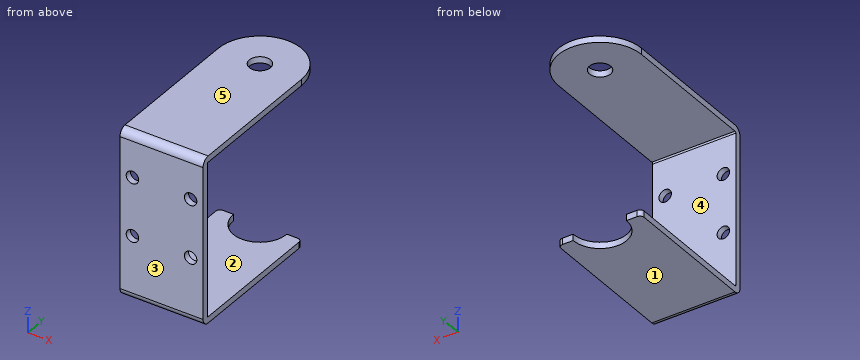
Autodesk Inventor part; units mm, degrees
ref_plane "YZ Plane" through (0, 0, 0) normal (1, 0, 0) x (0, 1, 0)
ref_plane "XZ Plane" through (0, 0, 0) normal (0, 1, 0) x (-1, 0, 0)
ref_plane "XY Plane" through (0, 0, 0) normal (0, 0, 1) x (1, 0, 0)
sketch "Sketch1" plane through (0, 0, 0) normal (0, 1, 0) x (-1, 0, 0)
  line L0 (10, -18.5) -> (-10, -18.5)
  line L1 (-10, -18.5) -> (-10, 18.5)
  line L2 (-10, 18.5) -> (10, 18.5)
  line L3 (10, 18.5) -> (10, -18.5)
  point P0 (0, 0)
  dimension "d0" = 20
  dimension "d1" = 37
  dimension "d2" = 18.5
  dimension "d3" = 10
extrude "Plate1" add sketch "Sketch1" along normal blind 1.5
sketch "Sketch2" plane through (-10, 0, -20) normal (0, 0, 1) x (1, 0, 0)
  line L0 (20, 0) -> (0, 0)
  line L1 (0, 0) -> (0, 45.1)
  line L2 (0, 45.1) -> (20, 45.1)
  line L3 (20, 45.1) -> (20, 0)
edge flange "Flange1" height 45.1 angle 90 thickness 1.5 bend radius 0.31 thickness toward (0, 0, 1) relief tear relief width 1.5 relief depth 0.75 edges at (0, 1.5, -18.5) wall of the first edge with corners at (10, 0, -20) (-10, 0, -20) (-10, 45.1, -20) (10, 45.1, -20)
bend "Bend1"
corner "Corner1"
sketch "Sketch3" plane through (10, 0, 20) normal (0, 0, -1) x (-1, 0, 0)
  line L0 (20, 0) -> (0, 0)
  line L1 (0, 0) -> (0, 45.1)
  line L2 (0, 45.1) -> (20, 45.1)
  line L3 (20, 45.1) -> (20, 0)
edge flange "Flange2" height 45.1 angle 90 thickness 1.5 bend radius 0.31 thickness toward (0, 0, -1) relief tear relief width 1.5 relief depth 0.75 edges at (0, 1.5, 18.5) wall of the first edge with corners at (-10, 0, 20) (10, 0, 20) (10, 45.1, 20) (-10, 45.1, 20)
bend "Bend2"
corner "Corner2"
sketch "Sketch4" plane through (-10, 45.1, 20) normal (0, 0, 1) x (1, 0, 0)
  circle A0 centre (10, -10) radius 10
  line L0 (0, 0) -> (20, 0)
  line L1 (0, 0) -> (20, 0)
  line L2 (20, 0) -> (20, -10)
  line L3 (20, -10) -> (0, -10)
  line L4 (0, -10) -> (0, 0)
  line L5 (0, -43.29) -> (0, 0)
  point P0 (10, -45.1)
  point P1 (10, -10)
  point P2 (20, 0)
  point P3 (10, 0)
  point P4 (0, -10)
  point P5 (8.5893, 0)
  point P6 (0, -10)
  dimension "d26" = 20
  dimension "d25" = 10
  dimension "d27" = 10
  dimension "d28" = 10
extrude "Extrusion1" cut sketch "Sketch4" against normal blind 10 contours L4 L0 A0 | A0 L0 L2
sketch "Sketch5" plane through (10, 45.1, -20) normal (0, 0, -1) x (-1, 0, 0)
  arc A0 (20, -10) -> (0, -10) centre (10, -10) ccw
  point P0 (10, -45.1)
hole "Hole1" at (0, 35.1, -20) direction (0, 0, 1) diameter 12.8 depth 1.5
sketch "Sketch6" plane through (10, 45.1, -20) normal (0, 0, -1) x (-1, 0, 0)
  circle A0 centre (10, -10) radius 6.4
  line L0 (0, 0) -> (20, 0)
  line L1 (0, -43.29) -> (0, 0)
  line L2 (24, 0) -> (-4, 0)
  line L3 (-4, 0) -> (-4, -9.9)
  line L4 (-4, -9.9) -> (24, -9.9)
  line L5 (24, -9.9) -> (24, 0)
  point P0 (10, -45.1)
  point P1 (20, 0)
  point P2 (6.005, 0)
  point P3 (13.995, 0)
  dimension "d38" = 9.9
  dimension "d39" = 4
  dimension "d40" = 28
extrude "Extrusion2" cut sketch "Sketch6" against normal blind 10 contours L4 A0 | A0 L4 L1 L0 L2 L5 | L4 L3 L2 L1 picked at (9.1972, -6.4205)
fillet "Fillet1" radius 1 2 edges at (-10, 35.2, -19.25) (10, 35.2, -19.25)
sketch "Sketch7" plane through (-10, 1.81, 20) normal (0, 0, 1) x (1, 0, 0)
  arc A0 (20, 33.29) -> (0, 33.29) centre (10, 33.29) ccw
  point P0 (10, -1.81)
hole "Hole2" at (0, 35.1, 20) direction (0, 0, -1) diameter 5.1 depth 1.5
sketch "Sketch8" plane through (0, 0, 0) normal (0, -1, 0) x (1, 0, 0)
  line L0 (2.55, 18.5) -> (-2.55, 18.5)
  line L1 (-10, 18.5) -> (10, 18.5)
  line L2 (10, 18.5) -> (-10, 18.5)
  line L3 (10, 18.19) -> (-10, 18.19)
  line L4 (-10, -18.19) -> (-10, 18.19)
  line L5 (-10, -18.19) -> (10, -18.19)
  line L6 (10, 18.19) -> (10, -18.19)
  point P0 (0, 0)
  point P1 (7, 9.5)
  point P2 (7, -4.5)
  point P3 (-7, 9.5)
  point P4 (-7, -4.5)
  dimension "d51" = 9
  dimension "d52" = 3
  dimension "d55" = 14
  dimension "d58" = 14
hole "Hole3" at (7, 0, 9.5) at (7, 0, -4.5) at (-7, 0, 9.5) at (-7, 0, -4.5) direction (0, 1, 0) diameter 3 depth 1.5
equation "\"d36\" = Thickness"
equation "\"d49\" = Thickness"
equation "\"d66\" = Thickness"
equation "\"d4\" = Thickness"
equation "\"d5\" = BendReliefWidth"
equation "\"d6\" = BendReliefDepth"
equation "\"d7\" = MinimumRemnant"
equation "\"d8\" = TransitionRadius"
equation "\"d11\" = BendRadius"
equation "\"d12\" = CornerReliefSize"
equation "\"d13\" = GapSize"
equation "\"d14\" = JacobiRadiusSize"
equation "\"d15\" = BendReliefWidth"
equation "\"d16\" = BendReliefDepth"
equation "\"d17\" = MinimumRemnant"
equation "\"d18\" = TransitionRadius"
equation "\"d21\" = BendRadius"
equation "\"d22\" = CornerReliefSize"
equation "\"d23\" = GapSize"
equation "\"d24\" = JacobiRadiusSize"
equation "\"BendReliefWidth\" = Thickness"
equation "\"BendReliefDepth\" = 0.5 * Thickness"
equation "\"CornerReliefSize\" = 4 * Thickness"
equation "\"MinimumRemnant\" = 2 * Thickness"
equation "\"TransitionRadius\" = BendRadius"
equation "\"JacobiRadiusSize\" = BendRadius"
equation "\"GapSize\" = Thickness"
properties part number "axis_9_bottom_frame" material "Aluminum 6061-AHC"
CAD build for the part. Positions are in the model's coordinates, mm. Face numbers are marked on the shaded views. A direction names the side the tool comes from. Coordinates: 2 decimals unless noted, no trailing zeros. Order: outer loops, then holes, each group sorted by start corner. A loop starts at its lowest first (then second) coordinate and runs counter-clockwise, first axis right, second up. Notation, with made-up numbers: (87, -27.5) -> (138, -27.5) arc R18 ccw to (138, 7.5) -> close; hole circle Ø8 at (-19, -25). An arc over 180 degrees is marked (long way). Use one line per item in the form item = value. Start each with the question number.
1) Band-saw the part on B-B on y = 5.5. Give the cut face in (x, z).
2) Tool access for the marked faces 1 and 2: list every direction of +Z, -Z, +X, -X, +Y, -Y with a clear straight run to the whole face (end or side of a thin tool).
3) Band-saw the part on A-A on z = -4.5. Give the cut face in (x, y).
4) Band-saw the part on C-C on x = 0. Give the cut face in (y, z), then the cut area to 3 significant figures.
5) Pull direction Z, two halves, no side cores. Call the marked faces 3, 4 and 5: +Z half, -Z half, draft (parallel to the pull), parting line (faces both ways), or undercut.
6) Drop flat-ended pins along their axis: pin 1 (1.5 mm diameter, centred on x = 7, z = 14, fed in from +Y); pin 2 (3 mm diameter, centred on x = -1.5, y = 39, fed in from -Z); pin 3 (2.5 mm diameter, centred on x = -7, z = 9.5, fed in from -Y); pin 4 (0.8 mm diameter, centred on x = -7, z = -19.5, fed in from +Y). Give the stop position or say it passes through.
7) Drill centre lines: L1, parallel to X at y = 0.9, z = -4.5; L2, parallel to Z at x = 0.5, y = 17.5; L3, parallel to Z at x = 7, y = 0.9. Where is each one in solid material? Low to high. Write a range as [from, to].
8) Band-saw the part on D-D on x = 7. Give the cut face in (y, z).
Entries:
q1.outline = (-10, -20) -> (10, -20) -> (10, -18.5) -> (-10, -18.5) -> close; (-10, 18.5) -> (10, 18.5) -> (10, 20) -> (-10, 20) -> close
q2.face_1 = -Z, +X, -X, +Y, -Y
q2.face_2 = +X, -X, +Y
q3.outline = (-10, 0) -> (-8.5, 0) -> (-8.5, 1.5) -> (-10, 1.5) -> close; (-5.5, 0) -> (5.5, 0) -> (5.5, 1.5) -> (-5.5, 1.5) -> close; (8.5, 0) -> (10, 0) -> (10, 1.5) -> (8.5, 1.5) -> close
q4.outline = (0, -18.19) arc R1.81 ccw to (1.81, -20) -> (28.7, -20) -> (28.7, -18.5) -> (1.81, -18.5) arc R0.31 cw to (1.5, -18.19) -> (1.5, 18.19) arc R0.31 cw to (1.81, 18.5) -> (32.55, 18.5) -> (32.55, 20) -> (1.81, 20) arc R1.81 ccw to (0, 18.19) -> close; (37.65, 18.5) -> (45.1, 18.5) -> (45.1, 20) -> (37.65, 20) -> close
q4.area = 157 mm2
q5.face_3 = draft
q5.face_4 = undercut
q5.face_5 = +Z half
q6.pin_1 = 1.5
q6.pin_2 = 18.5
q6.pin_3 = through
q6.pin_4 = 35.2
q7.L1 = [-10, -8.5], [-5.5, 5.5], [8.5, 10]
q7.L2 = [-20, -18.5], [18.5, 20]
q7.L3 = [-19.75, -6], [-3, 8], [11, 19.75]
q8.outline = (0, -18.19) arc R1.81 ccw to (1.81, -20) -> (35.2, -20) -> (35.2, -18.5) -> (1.81, -18.5) arc R0.31 cw to (1.5, -18.19) -> (1.5, -6) -> (0, -6) -> close; (0, -3) -> (1.5, -3) -> (1.5, 8) -> (0, 8) -> close; (0, 11) -> (1.5, 11) -> (1.5, 18.19) arc R0.31 cw to (1.81, 18.5) -> (42.24, 18.5) -> (42.24, 20) -> (1.81, 20) arc R1.81 ccw to (0, 18.19) -> close
